Design review of the part built by this model. Coordinates are the model's own, in mm. Face numbers are marked on the shaded views. Give positions to 0.01 mm unless a question says otherwise; leave off trailing zeros. Loops run counter-clockwise (first coordinate to the right, second up) from the corner with the lowest first, then second, coordinate; pieces in that order, holes last. Notation, with made-up numbers: (21, 79) -> (52, 79) arc R18 ccw to (52, 102) -> close; hole circle Ø9 at (3.25, 17.25). An arc over 180 degrees is marked (long way). Use a Markdown table: item, result. Add a question column.
1. Add section B-B (x = 0). Count the separate pieces of the cut face and the enclosed holes in it, and give its area (3 significant figures).
2. For pin 1 Ø6 at (x, z) = (28.5, -6) entering from -Y; pin 2 Ø6 at (x, z) = (-62, -6) entering from -Y; pin 3 Ø12.5 at (x, y) = (52.09, 0) entering from -Z; pin 4 Ø6 at (y, z) = (5, -1.5) entering from +X (3 decimals), all flat-tipped, find the tip position at first contact; note any pin that passes through.
3. Draft analysis for pull direction Y (two halves, no side actions). For the marked faces 1, 2 and 3, state which applies: pulls with the +Y half, pulls with the -Y half, needs draft (parallel to the pull), parting line crosses it, or undercut.
4. To check wall thickness, follow line 1 (Y direction, x = 0, z = -5.5); line 2 (X direction, y = -9, z = -2.5); line 3 (X direction, y = 64, z = -1.25). State the ranges of each line that lie inside material, in increasing order.
5. Add section A-A (y = 0). State the section outline as (x, z) points.
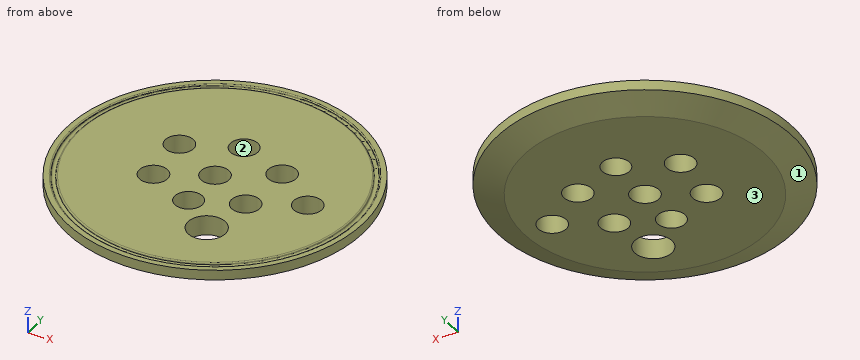
```python
from build123d import *

# Parameters (mm, degrees)
SKETCH2_R          = 7.9375
SKETCH2_R_2        = 7.75
SKETCH2_R_3        = 10.5
CUT_EXTRUDE1_DEPTH = 119.521470637


with BuildPart() as part:
    # Sketch1 → Revolve1 (revolve)
    with BuildSketch(Plane(origin=(0, 0, 0), x_dir=(0, 0, -1), z_dir=(1, 0, 0)), mode=Mode.PRIVATE) as revolve1_sk:
        with BuildLine():
            Line((0, 0), (0, 76.444627725))
            ThreePointArc((0, 76.444627725), (0.130798304, 76.879222907), (0.479738309, 77.169433247))
            Line((0.479738309, 77.169433247), (0.872854821, 77.336301306))
            ThreePointArc((0.872854821, 77.336301306), (1.6002, 78.4352), (0.872854821, 79.534098694))
            Line((0.872854821, 79.534098694), (0.479738309, 79.700966753))
            ThreePointArc((0.479738309, 79.700966753), (0.130798304, 79.991177093), (0, 80.425772275))
            Line((0, 80.425772275), (0, 83.439))
            Line((0, 83.439), (5.588, 83.439))
            Line((5.588, 83.439), (11.0998, 68.295453959))
            Line((11.0998, 68.295453959), (11.0998, 0))
            Line((11.0998, 0), (0, 0))
        make_face()
    revolve(revolve1_sk.sketch.rotate(Axis((0, 0, 0), (0, 0, -1)), 90), axis=Axis((0, 0, 0), (0, 0, -1)))

    # Sketch2 → Cut-Extrude1 (cut, through all)
    with BuildSketch(Plane(origin=(0, 0, -11.0998), x_dir=(-1, 0, 0), z_dir=(0, 0, -1))):
        Circle(SKETCH2_R)
        with Locations((0, 27.9765569)):
            Circle(SKETCH2_R_2)
        with Locations((-25.552434697, -14.308394833)):
            Circle(SKETCH2_R)
        with Locations((-52.091958056, 0)):
            Circle(SKETCH2_R)
        with Locations((26.222693633, -14.308394833)):
            Circle(SKETCH2_R)
        with Locations((-27.556050936, 17.333644944)):
            Circle(SKETCH2_R)
        with Locations((28.655279996, 14.787165533)):
            Circle(SKETCH2_R)
        with Locations((0, -25.424326978)):
            Circle(SKETCH2_R_2)
        with Locations((-19.725243494, -41.754750634)):
            Circle(SKETCH2_R_3)
    extrude(amount=-CUT_EXTRUDE1_DEPTH, mode=Mode.SUBTRACT)


solid = part.part
```
Taken from the geometry:
| question | item | result |
|---|---|---|
| 1 | separate pieces | 4 |
| 1 | enclosed holes | 0 |
| 1 | area | 1,240 mm^2 |
| 2 | pin 1 | stops at y = -79.44 |
| 2 | pin 2 | stops at y = -58.97 |
| 2 | pin 3 | passes through |
| 2 | pin 4 | stops at x = 83.415 |
| 3 | face 1 | parting line crosses it |
| 3 | face 2 | undercut |
| 3 | face 3 | needs draft |
| 4 | line 1 | y = -83.44 to -33.17, -17.67 to -7.94, 7.94 to 20.23, 35.73 to 83.44 |
| 4 | line 2 | x = -82.95 to -32.12, -20.32 to 19.65, 31.45 to 82.95 |
| 4 | line 3 | x = -53.54 to -46.79, -43.87 to 43.87, 46.79 to 53.54 |
| 5 | outline | (-83.44, -5.59) -> (-68.3, -11.1) -> (-7.94, -11.1) -> (-7.94, 0) -> (-76.44, 0) arc R0.79 ccw to (-77.17, -0.48) -> (-77.34, -0.87) arc R1.19 cw to (-79.53, -0.87) -> (-79.7, -0.48) arc R0.79 ccw to (-80.43, 0) -> (-83.44, 0) -> close; (7.94, -11.1) -> (44.15, -11.1) -> (44.15, 0) -> (7.94, 0) -> close; (60.03, -11.1) -> (68.3, -11.1) -> (83.44, -5.59) -> (83.44, 0) -> (80.43, 0) arc R0.79 ccw to (79.7, -0.48) -> (79.53, -0.87) arc R1.19 cw to (77.34, -0.87) -> (77.17, -0.48) arc R0.79 ccw to (76.44, 0) -> (60.03, 0) -> close |
